```python
from build123d import *

# Parameters (mm, degrees)
F1_DEPTH = 41.275
F0_W     = 42.8625
F0_H     = 117.475
F2_DEPTH = 30.1625
F0_W_2   = 12.7
F3_DEPTH = 41.275
F0_R     = 10.31875
F4_DEPTH = 17.4625


with BuildPart() as f1:
    # F0 (on Top) → F1 (new body)
    with BuildSketch(Plane.XY):
        Polygon((-1.5875, -58.7375), (11.1125, -58.7375), (11.1125, 58.7375), (-1.5875, 58.7375), (-1.5875, 4.7625), align=None)
    extrude(amount=F1_DEPTH)

    # F0 (on Top) → F2 (join)
    with BuildSketch(Plane.XY):
        with Locations((32.54375, 0)):
            Rectangle(F0_W, F0_H)
    extrude(amount=F2_DEPTH)

    # F0 (on Top) → F3 (join)
    with BuildSketch(Plane.XY):
        with Locations((60.325, 0)):
            Rectangle(F0_W_2, F0_H)
    extrude(amount=F3_DEPTH)

    # F0 (on Top) → F4 (join)
    with BuildSketch(Plane.XY):
        Polygon((-66.675, -58.7375), (-1.5875, -58.7375), (-1.5875, 4.7625), (-1.5875, 58.7375), (-66.675, 58.7375), align=None)
        with Locations((-34.925, -26.9875)):
            Circle(F0_R, mode=Mode.SUBTRACT)
        with Locations((-34.925, 36.5125)):
            Circle(F0_R, mode=Mode.SUBTRACT)
    extrude(amount=F4_DEPTH)


solid = f1.part
```
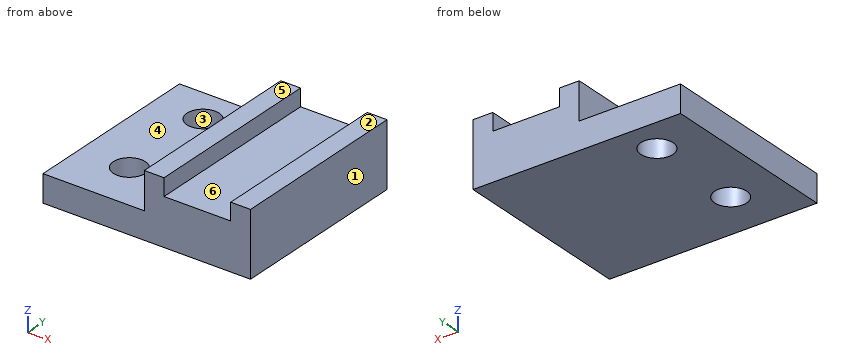
Here's how the part is built. I have some questions about the finished solid (model axes, mm). Face numbers are marked on the shaded views. A direction names the side the tool comes from. Coordinates: 2 decimals unless noted, no trailing zeros. Write each loop counter-clockwise with the first axis right and the second up, starting at its lowest first coordinate (ties: lowest second). Pieces come first, ordered by that corner, then holes. Notation, with made-up numbers: (8.5, -19) -> (42.5, -19) arc R24 cw to (42.5, 14) -> close; hole circle Ø9 at (31.5, 14). An arc over 180 degrees is marked (long way). Use a Markdown table: item, result. Add a question column.
(1) Please list where these lines run through material, in increasing order: line 1 (X direction, y = -17.5, z = 30.5) (1 decimal); line 2 (Y direction, x = -28, z = 12.5); line 3 (X direction, y = -5.5, z = 30) (1 decimal).
(2) If we section it at D-D, the plane z = 8.5: Write out the boundary of the cut face in (x, y) (1 decimal).
(3) For the marked faces 4, 5 and 6, which set-ups out of +Z, -Z, +X, -X, +Y, -Y let a thin tool reach every point of the face, with its end or its side?
(4) We'd pull the mould along X, two halves only. Please class the marked faces 1, 2 and 3: +X half, -X half, draft (parallel to the pull), parting line (faces both ways), or undercut.
(5) I'm going to push flat-ended pins straight in: P1, Ø16.5, axis at x = -34.92, y = -26.99, coming from the -Z side; P2, Ø10, axis at x = 21.5, y = -39.5, coming from the -Z side; P3, Ø5, axis at x = 42, y = -29, coming from the +Z side; P4, Ø12, axis at y = 15, z = 34, coming from the -X side. Where does each tip first touch, or does it pass through?
(6) If we section it at B-B, the plane z = 36.5: Write out the boundary of the cut face in (x, y) (1 decimal).
(7) If we section it at A-A, the plane y = -32: Write out the boundary of the cut face in (x, z) (1 decimal), and give its area (3 significant figures).
(8) If we section it at C-C, the plane y = 12: Write out the boundary of the cut face in (x, z) (1 decimal), and give its area (3 significant figures).
Outcome:
| question | item | result |
|---|---|---|
| 1 | line 1 | x = -1.6 to 11.1, 54 to 66.7 |
| 1 | line 2 | y = -58.74 to -34.64, -19.34 to 28.86, 44.16 to 58.74 |
| 1 | line 3 | x = -1.6 to 66.7 |
| 2 | outline | (-66.7, -58.7) -> (66.7, -58.7) -> (66.7, 58.7) -> (-66.7, 58.7) -> close; hole circle Ø20.6 at (-34.9, -27); hole circle Ø20.6 at (-34.9, 36.5) |
| 3 | face 4 | +Z, -X, +Y, -Y |
| 3 | face 5 | +Z, +X, -X, +Y, -Y |
| 3 | face 6 | +Z, +Y, -Y |
| 4 | face 1 | +X half |
| 4 | face 2 | draft |
| 4 | face 3 | undercut |
| 5 | P1 | passes through |
| 5 | P2 | stops at z = 0 |
| 5 | P3 | stops at z = 30.16 |
| 5 | P4 | stops at x = -1.59 |
| 6 | outline | (-1.6, -58.7) -> (11.1, -58.7) -> (11.1, 58.7) -> (-1.6, 58.7) -> close; (54, -58.7) -> (66.7, -58.7) -> (66.7, 58.7) -> (54, 58.7) -> close |
| 7 | outline | (-66.7, 0) -> (-43.9, 0) -> (-43.9, 17.5) -> (-66.7, 17.5) -> close; (-25.9, 0) -> (66.7, 0) -> (66.7, 41.3) -> (54, 41.3) -> (54, 30.2) -> (11.1, 30.2) -> (11.1, 41.3) -> (-1.6, 41.3) -> (-1.6, 17.5) -> (-25.9, 17.5) -> close |
| 7 | area | 3,160 mm^2 |
| 8 | outline | (-66.7, 0) -> (66.7, 0) -> (66.7, 41.3) -> (54, 41.3) -> (54, 30.2) -> (11.1, 30.2) -> (11.1, 41.3) -> (-1.6, 41.3) -> (-1.6, 17.5) -> (-66.7, 17.5) -> close |
| 8 | area | 3,480 mm^2 |
